Here's the drawing with two shaded views (mm, measured from the low corner). I have some questions. A direction names the side the tool comes from. Round coordinates to 2 decimals unless told otherwise and drop trailing zeros. Loops run counter-clockwise (first coordinate to the right, second up) from the corner with the lowest first, then second, coordinate; pieces in that order, holes last.
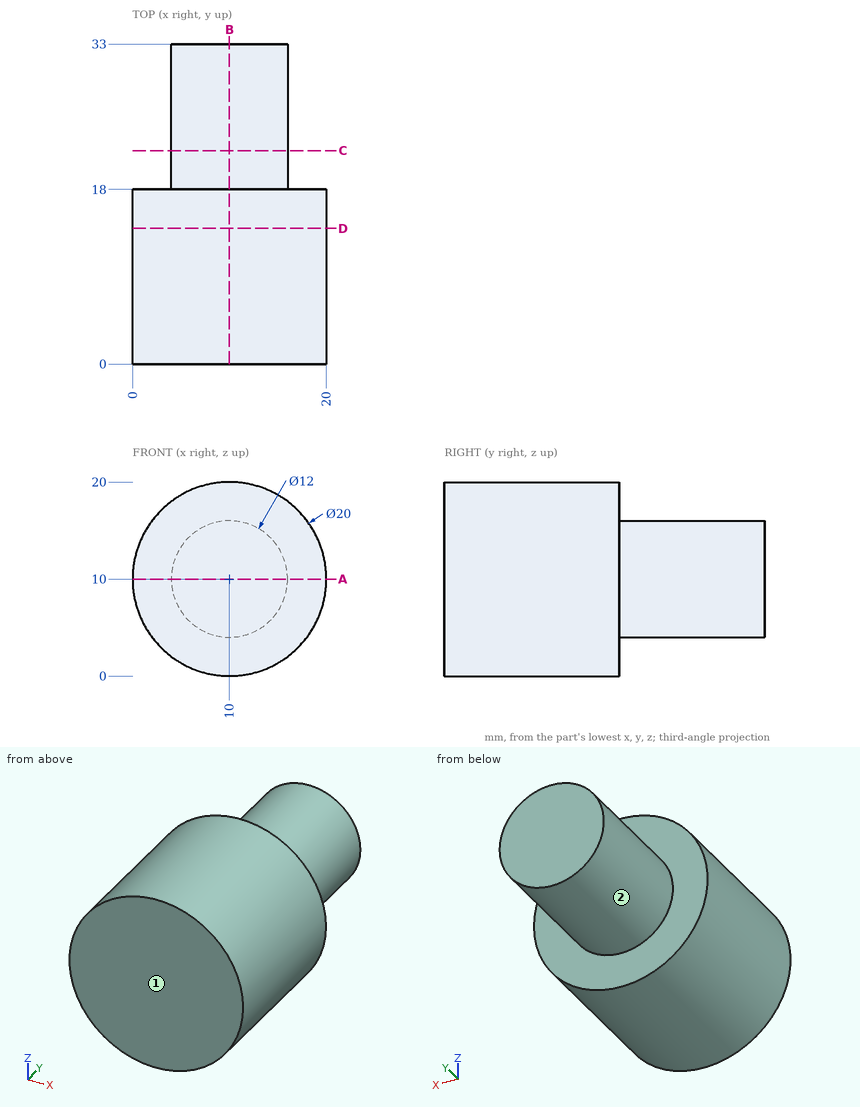
Item 1: If we section it at C-C, the plane y = 22: Please give me the cut outline in (x, z).
Results list:
outline: circle Ø12 at (10, 10)
Item 2: If I drill on line 1 along Y through (x, z) = (2.5, 12); line 2 along X through (y, z) = (7, 10.25), over which ranges is the centre line in solid material (lowest first)?
Results list:
line 1: y = 0 to 18
line 2: x = 0 to 20
Item 3: For the marked faces 1 and 2, which set-ups out of +Z, -Z, +X, -X, +Y, -Y let a thin tool reach every point of the face, with its end or its side?
Results list:
face 1: +Z, -Z, +X, -X, -Y
face 2: +Y
Item 4: If we section it at D-D, the plane y = 14: Please give me the cut outline in (x, z), then the cut area to 3 significant figures.
Results list:
outline: circle Ø20 at (10, 10)
area: 314 mm2
Item 5: If we section it at A-A, the plane z = 10: Please give me the cut outline in (x, y), then the cut area to 3 significant figures.
Results list:
outline: (0, 0) - (20, 0) - (20, 18) - (16, 18) - (16, 33) - (4, 33) - (4, 18) - (0, 18) - close
area: 540 mm2
Item 6: Will these pins go through, and if not, where does the flat tip stop? pin 1 (12 mm diameter, centred on x = 3, y = 25.5, fed in from -Z); pin 2 (1.5 mm diameter, centred on x = 9.5, y = 24.5, fed in from +Z); pin 3 (1 mm diameter, centred on x = 4.5, z = 5.5, fed in from +Y).
Results list:
pin 1: stops at z = 4.08
pin 2: stops at z = 16
pin 3: stops at y = 18
Item 7: If we section it at B-B, the plane x = 10: Please give me the cut outline in (y, z), then the cut area to 3 significant figures.
Results list:
outline: (0, 0) - (18, 0) - (18, 4) - (33, 4) - (33, 16) - (18, 16) - (18, 20) - (0, 20) - close
area: 540 mm2
